Read the model definition and answer for the solid it produces. Units are mm, in the model's axes. A direction names the side the tool comes from. Coordinates: 2 decimals unless noted, no trailing zeros. Write each loop counter-clockwise with the first axis right and the second up, starting at its lowest first coordinate (ties: lowest second). Pieces come first, ordered by that corner, then holes. Notation, with made-up numbers: (53, 78.25) -> (59, 78.25) arc R25 ccw to (59, 112.25) -> close; hole circle Ø8 at (-33.75, -32). An arc over 180 degrees is marked (long way). Answer in a Markdown table with one row per item. Add a question column.
Item 1: Section B-B on x = 50 is taken. Write down the section's boundary in (y, z), then the cut area to 3 significant figures.
Item 2: Section D-D on y = -80 is taken. Write down the section's boundary in (x, z).
Item 3: Which of the six approach directions +Z, -Z, +X, -X, +Y, -Y give full straight-line access (tool end or side, diameter ignored) to faces 1 (the face through (10, -324, 54)), 2 (the face through (51.139, -288.676, 5.07))?
Item 4: Section A-A on z = 55 is taken. Write down the section's boundary in (x, y), then the cut area to 3 significant figures.
Item 5: For a pull along Y with two mould halves and no side action, classify faces 3 (the face through (0, -324, 51)), 4 (the face through (51.9, -471.46, 5.07)), 5 (the face through (5, -614, 54)), 6 (the face through (4.93, -388.346, 57.628)) as +Y half, -Y half, draft (parallel to the pull), parting line (faces both ways), or undercut.
Item 6: Section C-C on y = -180 is taken. Write down the section's boundary in (x, z), then the cut area to 3 significant figures.
Item 7: Given pin 1 Ø23 at (x, y) = (50, -380) entering from +Z, flat-ended and moving along its own axis, determine where the tip first touches the part or whether it passes through.
Item 8: Straight lines are drawn through the part: line 1 (X direction, y = -280, z = 3); line 2 (Z direction, x = 2, y = -380); line 3 (X direction, y = -76.5, z = 59). For each, find the intervals that lie inside material, in ascending order. Write a range as from..to.
```python
from build123d import *

# Parameters (mm, degrees)
F1_DEPTH = 658
F3_D     = 17.5
F5_D     = 17.5
F7_SIZE  = 90
F8_R     = 5


with BuildPart() as f1:
    # F0 (on Front) → F1 (new body)
    with BuildSketch(Plane.XZ):
        Polygon((0, 100), (0, 0), (100, 0), (100, 10), (10, 10), (10, 100), align=None)
    extrude(amount=F1_DEPTH)

    # F3 (through all)
    with Locations(Plane.YZ.offset(10)):
        with Locations((-180, 55), (-280, 55), (-380, 55), (-480, 55)):
            Hole(F3_D / 2)

    # F5 (through all)
    with Locations(Plane(origin=(0, 0, 0), x_dir=(1, 0, 0), z_dir=(0, 0, -1))):
        with Locations((50, 580), (50, 480), (50, 380), (50, 280), (50, 180), (50, 80)):
            Hole(F5_D / 2)

    # F7
    f7_edges = [f1.edges().sort_by_distance(p)[0] for p in [
        (5, -658, 100),
        (5, 0, 100),
    ]]
    chamfer(f7_edges, length=F7_SIZE)

    # F8
    f8_edges = [f1.edges().sort_by_distance(p)[0] for p in [
        (5, -90, 100),
        (100, 0, 5),
        (5, -568, 100),
        (100, -658, 5),
    ]]
    fillet(f8_edges, radius=F8_R)


solid = f1.part
```
Results below:
| question | item | result |
|---|---|---|
| 1 | outline | (-658, 0) -> (-588.75, 0) -> (-588.75, 10) -> (-658, 10) -> close; (-571.25, 0) -> (-488.75, 0) -> (-488.75, 10) -> (-571.25, 10) -> close; (-471.25, 0) -> (-388.75, 0) -> (-388.75, 10) -> (-471.25, 10) -> close; (-371.25, 0) -> (-288.75, 0) -> (-288.75, 10) -> (-371.25, 10) -> close; (-271.25, 0) -> (-188.75, 0) -> (-188.75, 10) -> (-271.25, 10) -> close; (-171.25, 0) -> (-88.75, 0) -> (-88.75, 10) -> (-171.25, 10) -> close; (-71.25, 0) -> (0, 0) -> (0, 10) -> (-71.25, 10) -> close |
| 1 | area | 5,530 mm2 |
| 2 | outline | (0, 0) -> (41.25, 0) -> (41.25, 10) -> (10, 10) -> (10, 90) -> (0, 90) -> close; (58.75, 0) -> (100, 0) -> (100, 10) -> (58.75, 10) -> close |
| 3 | face 1 | +Z, +X, +Y, -Y |
| 3 | face 2 | +Z, -Z |
| 4 | outline | (0, -613) -> (10, -613) -> (10, -488.75) -> (0, -488.75) -> close; (0, -471.25) -> (10, -471.25) -> (10, -388.75) -> (0, -388.75) -> close; (0, -371.25) -> (10, -371.25) -> (10, -288.75) -> (0, -288.75) -> close; (0, -271.25) -> (10, -271.25) -> (10, -188.75) -> (0, -188.75) -> close; (0, -171.25) -> (10, -171.25) -> (10, -45) -> (0, -45) -> close |
| 4 | area | 4,980 mm2 |
| 5 | face 3 | draft |
| 5 | face 4 | undercut |
| 5 | face 5 | -Y half |
| 5 | face 6 | undercut |
| 6 | outline | (0, 0) -> (41.25, 0) -> (41.25, 10) -> (10, 10) -> (10, 46.25) -> (0, 46.25) -> close; (0, 63.75) -> (10, 63.75) -> (10, 100) -> (0, 100) -> close; (58.75, 0) -> (100, 0) -> (100, 10) -> (58.75, 10) -> close |
| 6 | area | 1,550 mm2 |
| 7 | pin 1 | stops at z = 10 |
| 8 | line 1 | x = 0..41.25, 58.75..100 |
| 8 | line 2 | z = 0..46.25, 63.75..100 |
| 8 | line 3 | x = 0..10 |
